Verification items for the finished model (mm, model axes). A direction names the side the tool comes from. Round coordinates to 2 decimals unless told otherwise and drop trailing zeros. Write each loop counter-clockwise with the first axis right and the second up, starting at its lowest first coordinate (ties: lowest second). Pieces come first, ordered by that corner, then holes. Notation, with made-up numbers: (77, 29.25) - (127, 29.25) arc R24 ccw to (127, 48.25) - close; hole circle Ø1 at (41.25, 38.25). An arc over 180 degrees is marked (long way). Answer as a JSON object with one key per item and string values. Group by question number.
1) Section check B-B (z = 1.5). Enter the section's corners in (x, y).
2) Section check D-D (y = 19.25). Enter the section's corners in (x, z), then the cut area to 3 significant figures.
3) Section check C-C (y = 17). Enter the section's corners in (x, z).
4) Section check A-A (x = -12). Enter the section's corners in (y, z).
5) Thickness scan on line 1 (X direction, y = 19.5, z = 0); line 2 (X direction, y = 13, z = 0); line 3 (Z direction, x = -12, y = 14). Record the ranges inside material, lowest first.
6) Set-up check for faces 1 (the flat face through (-9, 11, 0)), 2 (the cylindrical face through (-4.291, 14.451, -5.715)), 3 (the flat face through (-3.99, 14, 0)), 4 (the cylindrical face through (-15.248, 15.437, 5.287)), 5 (the cylindrical face through (-4.275, 14.549, 5.699)): record each of +Z, -Z, +X, -X, +Y, -Y from which the full face is reachable in a straight line by a thin tool's end or side.
7) Go/stop test with flat-tipped pins: pin 1 Ø2 at (y, z) = (14, 2) entering from +X; pin 2 Ø1 at (x, z) = (9, 1.5) entering from -Y. Record where each tip stops, or that it passes through.
8) Mould release check, pull along Z, two halves, no side actions. Record for faces 6 (the cylindrical face through (-14.44, 15.44, -0.54)), 7 (the cylindrical face through (15.248, 18.986, -5.287)), 8 (the flat face through (16, 19, 0)), 9 (the cylindrical face through (9.56, 18.99, -0.54)): +Z half, -Z half, draft (parallel to the pull), parting line (faces both ways), or undercut.
```python
from build123d import *

# Parameters (mm, degrees)
SKETCH_1_R          = 2.5
EXTRUDE_1_DEPTH     = 20
SKETCH_2_W          = 28.6658273
SKETCH_2_H          = 20.338801826
CUT_EXTRUDE_1_DEPTH = 18
SKETCH_3_W          = 21.28696294
SKETCH_3_H          = 15.18623143
CUT_EXTRUDE_2_DEPTH = 11
FILLET_1_R          = 1


with BuildPart() as part:
    # Эскиз1 → Бобышка-Вытянуть1 (new body)
    with BuildSketch(Plane(origin=(0, 0, 0), x_dir=(1, 0, 0), z_dir=(0, 1, 0))):
        with BuildLine():
            Line((-13.5, 6), (13.5, 6))
            ThreePointArc((13.5, 6), (15.267766953, 5.267766953), (16, 3.5))
            Line((16, 3.5), (16, -3.5))
            ThreePointArc((16, -3.5), (15.267766953, -5.267766953), (13.5, -6))
            Line((13.5, -6), (-13.5, -6))
            ThreePointArc((-13.5, -6), (-15.267766953, -5.267766953), (-16, -3.5))
            Line((-16, -3.5), (-16, 3.5))
            ThreePointArc((-16, 3.5), (-15.267766953, 5.267766953), (-13.5, 6))
        make_face()
        with Locations(Location((-12, 0, 0), (0, 0, 270))):
            Circle(SKETCH_1_R, mode=Mode.SUBTRACT)
        with Locations(Location((12, 0, 0), (0, 0, 270))):
            Circle(SKETCH_1_R, mode=Mode.SUBTRACT)
    extrude(amount=EXTRUDE_1_DEPTH)

    # Эскиз2 → Вырез-Вытянуть1 (cut)
    with BuildSketch(Plane.XZ):
        with Locations((10.342984763, 0)):
            Rectangle(SKETCH_2_W, SKETCH_2_H)
    extrude(amount=-CUT_EXTRUDE_1_DEPTH, mode=Mode.SUBTRACT)

    # Эскиз3 → Вырез-Вытянуть2 (cut)
    with BuildSketch(Plane.XZ):
        with Locations((-5.752302283, -0.036989119)):
            Rectangle(SKETCH_3_W, SKETCH_3_H)
    extrude(amount=-CUT_EXTRUDE_2_DEPTH, mode=Mode.SUBTRACT)

    # Скругление1
    fillet_1_edges = [part.edges().sort_by_distance(p)[0] for p in [
        (-3.989928887, 14.5, -6),
        (-3.989928887, 14.5, 6),
    ]]
    fillet(fillet_1_edges, radius=FILLET_1_R)


solid = part.part
```
Returned:
{
 "1": {"outline": "(-16, 11) - (-14, 11) - (-14, 20) - (-16, 20) - close; (-10, 11) - (-3.99, 11) - (-3.99, 18) - (10, 18) - (10, 20) - (-10, 20) - close; (14, 18) - (16, 18) - (16, 20) - (14, 20) - close"},
 "2": {"outline": "(-16, -3.5) arc R2.5 ccw to (-13.5, -6) - (13.5, -6) arc R2.5 ccw to (16, -3.5) - (16, 3.5) arc R2.5 ccw to (13.5, 6) - (-13.5, 6) arc R2.5 ccw to (-16, 3.5) - close; hole circle Ø5 at (-12, 0); hole circle Ø5 at (12, 0)", "area": "339 mm2"},
 "3": {"outline": "(-16, -3.5) arc R2.5 ccw to (-13.5, -6) - (-4.99, -6) arc R1 ccw to (-3.99, -5) - (-3.99, 5) arc R1 ccw to (-4.99, 6) - (-13.5, 6) arc R2.5 ccw to (-16, 3.5) - close; hole circle Ø5 at (-12, 0)"},
 "4": {"outline": "(11, -6) - (20, -6) - (20, -2.5) - (11, -2.5) - close; (11, 2.5) - (20, 2.5) - (20, 6) - (11, 6) - close"},
 "5": {"line 1": "-16 to -14.5, -9.5 to 9.5, 14.5 to 16", "line 2": "-16 to -14.5, -9.5 to -3.99", "line 3": "-6 to -2.5, 2.5 to 6"},
 "6": {"face 1": "+Z, -Z, +X, -X, -Y", "face 2": "-Z, +X, -Y", "face 3": "+Z, -Z, +X, -Y", "face 4": "+Z, -X, +Y, -Y", "face 5": "+Z, +X, -Y"},
 "7": {"pin 1": "x = -3.99", "pin 2": "y = 18"},
 "8": {"face 6": "undercut", "face 7": "-Z half", "face 8": "draft", "face 9": "undercut"}
}
